Autodesk Inventor part; units mm, degrees
ref_plane "YZ Plane" through (0, 0, 0) normal (1, 0, 0) x (0, 1, 0)
ref_plane "XZ Plane" through (0, 0, 0) normal (0, 1, 0) x (-1, 0, 0)
ref_plane "XY Plane" through (0, 0, 0) normal (0, 0, 1) x (1, 0, 0)
sketch "スケッチ1" plane through (0, 0, 0) normal (1, 0, 0) x (0, 1, 0)
  line L0 (0, 0) -> (-1, 0)
  line L1 (-1, 0) -> (-1, 10)
  line L2 (-1, 10) -> (0, 10)
  line L3 (0, 10) -> (0, 0)
  line L4 (0, 0) -> (-10, 0)
  line L5 (-10, 0) -> (-10, 1)
  line L6 (-10, 1) -> (0, 1)
  line L7 (0, 1) -> (0, 0)
  point P0 (-1, 1)
  dimension "d0" = 1
  dimension "d1" = 10
  dimension "d2" = 10
  dimension "d3" = 1
extrude "押し出し1" add sketch "スケッチ1" along normal blind 130
sketch "スケッチ2" plane through (0, 0, 10) normal (0, 1, 0) x (1, 0, 0)
  line L0 (0, 10) -> (0, 0)
  line L1 (0, 10) -> (130, 10)
  line L2 (130, 10) -> (130, 0)
  point P0 (5, 5)
  point P1 (125, 5)
  dimension "d13" = 5
  dimension "d14" = 5
  dimension "d15" = 5
  dimension "d16" = 5
hole "穴1" at (5, 0, 5) at (125, 0, 5) direction (0, -1, 0) diameter 3.5 end through all
sketch "スケッチ3" plane through (0, -10, 0) normal (0, 0, -1) x (-1, 0, 0)
  line L0 (0, 0) -> (-130, 0)
  line L1 (-130, 0) -> (-130, 10)
  line L2 (0, 0) -> (0, 10)
  point P0 (-115, 5)
  point P1 (-15, 5)
  dimension "d24" = 5
  dimension "d25" = 5
  dimension "d26" = 15
  dimension "d27" = 15
hole "穴2" at (115, -5, 0) at (15, -5, 0) direction (0, 0, 1) diameter 3.5 end through all
properties part number "slide_panel_joint"
Geometry: final body of the model. Coordinates: model frame, mm. A direction names the side the tool comes from. Round coordinates to 2 decimals unless told otherwise and drop trailing zeros. Order: outer loops, then holes, each group sorted by start corner. A loop starts at its lowest first (then second) coordinate and runs counter-clockwise, first axis right, second up. Notation, with made-up numbers: (-4, 31.5) -> (36, 31.5) arc R25 cw to (36, 59.5) -> close; hole circle Ø10 at (-7, 69). An arc over 180 degrees is marked (long way). Use one line per item in the form item = value.
(1) Section A-A on x = 5. Return loops of the section in (y, z).
Results list:
outline = (-10, 0) -> (0, 0) -> (0, 3.25) -> (-1, 3.25) -> (-1, 1) -> (-10, 1) -> close; (-1, 6.75) -> (0, 6.75) -> (0, 10) -> (-1, 10) -> close
(2) Access query for faces 4 (the face through (64, -5, 0)), 5 (the face through (64, -1, 5)). Directions: +Z, -Z, +X, -X, +Y, -Y. A direction counts if a zero-diameter tool reaches every point of the face in a straight line with its end or side. Return the directions, or none.
Results list:
face_4 = -Z, +X, -X, +Y, -Y
face_5 = +Z, +X, -X, -Y
(3) Section C-C on y = -5. Return loops of the section in (x, z).
Results list:
outline = (0, 0) -> (13.25, 0) -> (13.25, 1) -> (0, 1) -> close; (16.75, 0) -> (113.25, 0) -> (113.25, 1) -> (16.75, 1) -> close; (116.75, 0) -> (130, 0) -> (130, 1) -> (116.75, 1) -> close
(4) Section D-D on x = 78.5. Return loops of the section in (y, z), and give its area (3 significant figures).
Results list:
outline = (-10, 0) -> (0, 0) -> (0, 10) -> (-1, 10) -> (-1, 1) -> (-10, 1) -> close
area = 19.0 mm^2
(5) Draft query along Y for faces 1 (the face through (126.71, -0.51, 4.62)), 2 (the face through (113.265, -5.228, 0.507)), 3 (the face through (64, 0, 5)). Return one class per face: pulls with the +Y half, pulls with the -Y half, needs draft (parallel to the pull), parting line crosses it, or undercut.
Results list:
face_1 = needs draft
face_2 = undercut
face_3 = pulls with the +Y half
(6) Ray query, probe 1 along X at (y, z) = (-5, 0.55); probe 2 along X at (y, z) = (-0.65, 5); probe 3 along Z at (x, y) = (5, -0.65). Return the intervals inside material, ascending. Write a range as [from, to].
Results list:
probe_1 = [0, 13.25], [16.75, 113.25], [116.75, 130]
probe_2 = [0, 3.25], [6.75, 123.25], [126.75, 130]
probe_3 = [0, 3.25], [6.75, 10]
(7) Section B-B on z = 5. Return loops of the section in (x, y).
Results list:
outline = (0, -1) -> (3.25, -1) -> (3.25, 0) -> (0, 0) -> close; (6.75, -1) -> (123.25, -1) -> (123.25, 0) -> (6.75, 0) -> close; (126.75, -1) -> (130, -1) -> (130, 0) -> (126.75, 0) -> close
(8) First-contact query: pin 1 Ø4 at (x, z) = (64, 5.5) entering from -Y; pin 2 Ø2 at (x, y) = (15, -5) entering from -Z; pin 3 Ø4.5 at (x, y) = (115, -5) entering from +Z. Flat tips, straight axial feed; report the tip coordinate or a pass-through.
Results list:
pin_1 = -1
pin_2 = through
pin_3 = 1
